Geometry: final body of the model. Coordinates: model frame, mm. A direction names the side the tool comes from. Give positions to 0.01 mm unless a question says otherwise; leave off trailing zeros. Loops run counter-clockwise (first coordinate to the right, second up) from the corner with the lowest first, then second, coordinate; pieces in that order, holes last. Notation, with made-up numbers: (82.25, 75.5) -> (97.25, 75.5) arc R26 ccw to (97.25, 106.5) -> close; hole circle Ø5 at (1.5, -26). An arc over 180 degrees is marked (long way). Answer in a Markdown table with one row per item. Add a question column.
1) Section query B-B (z = 32). Return the cut outline in (x, y) (3 decimals).
2) First-contact query: P1, Ø16.5, axis at y = 40.5, z = 17, coming from the -X side; P2, Ø24.5, axis at x = 254, y = 25.4, coming from the +Z side (3 decimals); P3, Ø5.5, axis at x = 416.33, y = 23.91, coming from the -Z side (3 decimals). Flat tips, straight axial feed; report the tip coordinate or a pass-through.
3) Section query C-C (x = 368.3). Return the cut outline in (y, z) (3 decimals).
4) Line query: line 1 (Y direction, x = 402, z = 21) (3 decimals); line 2 (Z direction, x = 243.5, y = 11) (3 decimals). Output: solid intervals per line, ascending. Write a range as from..to.
5) Access query for faces 5 (the flat face through (25.4, 48, 18)), 6 (the cylindrical face through (501.982, 31.504, 49.235)), 7 (the flat face through (363, 8, 0)). Directions: +Z, -Z, +X, -X, +Y, -Y. A direction counts if a zero-diameter tool reaches every point of the face in a straight line with its end or side. Return the directions, or none.
6) Draft query along Z for faces 1 (the flat face through (736.6, 48, 22)), 2 (the flat face through (363, 9, 50.8)), 3 (the flat face through (376, 47.625, 26)), 4 (the flat face through (379, 3.175, 25)). Return one class per face: +Z half, -Z half, draft (parallel to the pull), parting line (faces both ways), or undercut.
7) Section query A-A (x = 556). Return the cut outline in (y, z) (3 decimals), plus the area to 3 significant figures.
Autodesk Inventor part; units mm, degrees
ref_plane "YZ Plane" through (0, 0, 0) normal (1, 0, 0) x (0, 1, 0)
ref_plane "XZ Plane" through (0, 0, 0) normal (0, 1, 0) x (-1, 0, 0)
ref_plane "XY Plane" through (0, 0, 0) normal (0, 0, 1) x (1, 0, 0)
sketch "Sketch1" plane through (0, 0, 0) normal (1, 0, 0) x (0, 1, 0)
  line L0 (0, 0) -> (50.8, 0)
  line L1 (50.8, 0) -> (50.8, 50.8)
  line L2 (50.8, 50.8) -> (0, 50.8)
  line L3 (0, 50.8) -> (0, 0)
  line L4 (3.175, 47.625) -> (47.625, 47.625)
  line L5 (47.625, 47.625) -> (47.625, 3.175)
  line L6 (47.625, 3.175) -> (3.175, 3.175)
  line L7 (3.175, 3.175) -> (3.175, 47.625)
  dimension "d0" = 50.8
  dimension "d1" = 3.175
extrude "Extrusion1" add sketch "Sketch1" along normal blind 736.6
sketch "Sketch2" plane through (0, 0, 50.8) normal (0, 0, 1) x (1, 0, 0)
  line L0 (0, 50.8) -> (0, 0)
  line L1 (0, 0) -> (736.6, 0)
  line L2 (736.6, 50.8) -> (736.6, 0)
  line L3 (0, 50.8) -> (736.6, 50.8)
  circle A0 centre (48.0624, 26.9875) radius 14.2875
  circle A1 centre (368.3, 23.8125) radius 14.2875
  circle A2 centre (688.5376, 26.9875) radius 14.2875
  line L4 (-35.152, 25.4) -> (810.7598, 25.4) construction
  line L5 (736.6, 3.175) -> (736.6, 0)
  line L6 (736.6, 0) -> (733.425, 0)
  arc A3 (733.425, 0) -> (736.6, 3.175) centre (733.425, 3.175) ccw
  arc A4 (0, 25.4) -> (1.4704, 22.7214) centre (3.175, 25.4) ccw
  arc A5 (36.3954, 0.4964) -> (38.1, 0) centre (38.1, 3.175) ccw
  line L7 (1.4704, 22.7214) -> (36.3954, 0.4964)
  line L8 (0, 25.4) -> (0, 0)
  line L9 (38.1, 0) -> (0, 0)
  line L10 (-134.201, 26.9875) -> (938.3775, 26.9875) construction
  dimension "d4" = 25.4
  dimension "d5" = 23.8125
  dimension "d6" = 320.2534
  dimension "d7" = 320.2534
  dimension "d8" = 368.3
  dimension "d9" = 28.575
  dimension "d10" = 3.175
  dimension "d11" = 3.175
  dimension "d12" = 3.175
  dimension "d13" = 3.175
  dimension "d14" = 38.1
  dimension "d19" = 1.5875
extrude "Extrusion2" cut sketch "Sketch2" against normal blind 50.8 contours A4 L7 A5 L1 L0 | L2 L1 A3 | A0 | A1 | A2
sketch "Sketch3" plane through (736.6, 50.8, 0) normal (0, 0, -1) x (-1, 0, 0)
  line L0 (736.6, 0) -> (711.2, 0)
  line L1 (711.2, 0) -> (711.2, -25.4)
  line L2 (711.2, -25.4) -> (736.6, -25.4)
  line L3 (736.6, -25.4) -> (736.6, 0)
  line L4 (711.2, -25.4) -> (717.8505, -18.7495) construction
  circle A0 centre (713.4451, -23.1549) radius 3.175
  point P0 (736.6, -50.8)
  dimension "d24" = 6.35
  dimension "d17" = 25.4
  dimension "d22" = 45
extrude "Extrusion3" cut sketch "Sketch3" against normal blind 47.625
sketch "Sketch5" plane through (0, 50.8, 50.8) normal (0, 0, 1) x (1, 0, 0)
  line L0 (0, 0) -> (736.6, 0)
  line L1 (0, 0) -> (0, -25.4)
  circle A0 centre (368.3, -26.9875) radius 14.2875
  line L2 (-82.8733, -25.4) -> (895.8965, -25.4) construction
  circle A1 centre (127, -25.4) radius 20.32
  circle A2 centre (254, -25.4) radius 20.32
  circle A3 centre (482.6, -25.4) radius 20.32
  circle A4 centre (609.6, -25.4) radius 20.32
  point P0 (0, -50.8)
  dimension "d25" = 25.4
  dimension "d26" = 40.64
  dimension "d27" = 127
  dimension "d28" = 127
  dimension "d29" = 114.3
  dimension "d30" = 114.3
extrude "Extrusion4" cut sketch "Sketch5" against normal blind 3.175 contours A1 | A2 | A3 | A4
sketch "Sketch6" plane through (733.425, 0, 0) normal (0, 0, -1) x (-1, 0, 0)
  line L0 (733.425, 25.4) -> (712.5151, 25.4)
  circle A0 centre (365.125, 23.8125) radius 14.2875
  line L1 (217.4406, 23.9141) -> (492.0781, 23.9141) construction
  point P0 (733.425, 0)
  point P1 (432.3588, 23.9141)
  point P2 (344.424, 23.9141)
  point P3 (317.0936, 23.9141)
  dimension "d33" = 0.1016
  dimension "d34" = 20.701
  dimension "d35" = 48.0314
  dimension "d36" = 67.2338
hole "Hole1" at (301.0662, 23.9141, 0) at (389.001, 23.9141, 0) at (416.3314, 23.9141, 0) direction (0, 0, 1) diameter 7.9756 depth 25.4 tip angle 118
sketch "Sketch7" plane through (733.425, 0, 0) normal (0, 0, -1) x (-1, 0, 0)
  line L0 (733.425, 25.4) -> (712.5151, 25.4)
  circle A0 centre (365.125, 23.8125) radius 14.2875
  line L1 (252.4125, 28.8925) -> (487.3625, 28.8925) construction
  point P0 (733.425, 0)
  point P1 (307.5686, 28.8925)
  point P2 (441.8838, 28.8925)
  dimension "d44" = 5.08
  dimension "d45" = 57.5564
  dimension "d46" = 76.7588
hole "Hole2" at (425.8564, 28.8925, 0) at (291.5412, 28.8925, 0) direction (0, 0, 1) diameter 6.35 depth 25.4 tip angle 118
sketch "Sketch8" plane through (0, 50.8, 50.8) normal (0, 0, 1) x (1, 0, 0)
  circle A0 centre (482.6, -25.4) radius 20.32
  circle A1 centre (127, -25.4) radius 20.32
  circle A2 centre (254, -25.4) radius 20.32
  circle A3 centre (609.6, -25.4) radius 20.32
  arc A4 (36.3954, -50.3036) -> (38.1, -50.8) centre (38.1, -47.625) ccw
  line L0 (38.1, -50.8) -> (733.425, -50.8)
  arc A5 (733.425, -50.8) -> (736.6, -47.625) centre (733.425, -47.625) ccw
  line L1 (736.6, 0) -> (736.6, -47.625)
  line L2 (0, 0) -> (736.6, 0)
  line L3 (0, 0) -> (0, -25.4)
  arc A6 (0, -25.4) -> (1.4704, -28.0786) centre (3.175, -25.4) ccw
  line L4 (1.4704, -28.0786) -> (36.3954, -50.3036)
  circle A7 centre (368.3, -26.9875) radius 14.2875
  circle A8 centre (48.0624, -23.8125) radius 14.2875
  circle A9 centre (688.5376, -23.8125) radius 14.2875
  circle A10 centre (291.5412, -21.9075) radius 3.175
  circle A11 centre (301.0662, -26.8859) radius 3.9878
  circle A12 centre (389.001, -26.8859) radius 3.9878
  circle A13 centre (416.3314, -26.8859) radius 3.9878
  circle A14 centre (425.8564, -21.9075) radius 3.175
  point P0 (0, -50.8)
hole "Hole3" at (301.0662, 23.9141, 50.8) at (389.001, 23.9141, 50.8) at (416.3314, 23.9141, 50.8) direction (0, 0, -1) diameter 4.7625 depth 25.4 tip angle 118
sketch "Sketch9" plane through (0, 50.8, 50.8) normal (0, 0, 1) x (1, 0, 0)
  circle A0 centre (291.5412, -21.9075) radius 3.175
  circle A1 centre (425.8564, -21.9075) radius 3.175
  point P0 (0, -50.8)
hole "Hole4" at (291.5412, 28.8925, 50.8) at (425.8564, 28.8925, 50.8) direction (0, 0, -1) diameter 9.525 depth 25.4 tip angle 118
sketch "Sketch11" plane through (733.425, 0, 0) normal (0, 0, -1) x (-1, 0, 0)
  circle A0 centre (307.5686, 28.8925) radius 3.175
  circle A1 centre (441.8838, 28.8925) radius 3.175
  circle A2 centre (344.424, 23.9141) radius 3.9878
  circle A3 centre (432.3588, 23.9141) radius 3.9878
  circle A4 centre (317.0936, 23.9141) radius 3.9878
  line L0 (708.025, 29.8901) -> (708.025, 50.8)
  line L1 (708.025, 50.8) -> (-3.175, 50.8)
  line L2 (-3.175, 3.175) -> (-3.175, 50.8)
  arc A5 (-3.175, 3.175) -> (0, 0) centre (0, 3.175) ccw
  line L3 (695.325, 0) -> (0, 0)
  arc A6 (695.325, 0) -> (697.0296, 0.4964) centre (695.325, 3.175) ccw
  line L4 (697.0296, 0.4964) -> (731.9546, 22.7214)
  arc A7 (731.9546, 22.7214) -> (733.425, 25.4) centre (730.25, 25.4) ccw
  line L5 (733.425, 25.4) -> (712.5151, 25.4)
  arc A8 (708.025, 29.8901) -> (712.5151, 25.4) centre (710.2701, 27.6451) ccw
  circle A9 centre (365.125, 23.8125) radius 14.2875
  circle A10 centre (685.3626, 26.9875) radius 14.2875
  circle A11 centre (44.8874, 26.9875) radius 14.2875
  point P0 (733.425, 0)
sketch "Sketch12" plane through (733.425, 0, 0) normal (0, 0, -1) x (-1, 0, 0)
  circle A0 centre (307.5686, 28.8925) radius 3.175
  circle A1 centre (441.8838, 28.8925) radius 3.175
  circle A2 centre (344.424, 23.9141) radius 3.9878
  circle A3 centre (432.3588, 23.9141) radius 3.9878
  circle A4 centre (317.0936, 23.9141) radius 3.9878
  line L0 (708.025, 29.8901) -> (708.025, 50.8)
  line L1 (708.025, 50.8) -> (-3.175, 50.8)
  line L2 (-3.175, 3.175) -> (-3.175, 50.8)
  arc A5 (-3.175, 3.175) -> (0, 0) centre (0, 3.175) ccw
  line L3 (695.325, 0) -> (0, 0)
  arc A6 (695.325, 0) -> (697.0296, 0.4964) centre (695.325, 3.175) ccw
  line L4 (697.0296, 0.4964) -> (731.9546, 22.7214)
  arc A7 (731.9546, 22.7214) -> (733.425, 25.4) centre (730.25, 25.4) ccw
  line L5 (733.425, 25.4) -> (712.5151, 25.4)
  arc A8 (708.025, 29.8901) -> (712.5151, 25.4) centre (710.2701, 27.6451) ccw
  circle A9 centre (365.125, 23.8125) radius 14.2875
  circle A10 centre (685.3626, 26.9875) radius 14.2875
  circle A11 centre (44.8874, 26.9875) radius 14.2875
  line L6 (713.7121, 11.1125) -> (756.5701, 38.3858)
  line L7 (733.425, 25.4) -> (733.425, 4.1402)
  line L8 (695.325, 0) -> (700.957, 0)
  line L9 (713.7121, 11.1125) -> (685.3626, -6.9281)
  line L10 (733.425, 23.6571) -> (740.2433, 12.9426)
  line L11 (696.2496, 0) -> (703.0679, -10.7145)
  line L12 (740.2433, 12.9426) -> (733.425, 12.9426)
  line L13 (703.0679, -10.7145) -> (703.0679, 0)
  line L14 (703.0679, 0) -> (696.2496, 0)
  point P0 (733.425, 0)
  dimension "d69" = 12.7
  dimension "d70" = 12.7
  dimension "d71" = 10.7145
  dimension "d72" = 6.8183
  dimension "d75" = 6.8183
  dimension "d76" = 37.1754
  dimension "d77" = 23.6571
equation "\"d7\" = d6"
equation "\"d11\" = d10"
equation "\"d13\" = d12"
equation "\"d28\" = d27"
equation "\"d30\" = d29"
properties part number "RightMainBeam" material "Aluminum 6061"
Evaluation:
| question | item | result |
|---|---|---|
| 1 | outline | (25.4, 47.625) -> (736.6, 47.625) -> (736.6, 50.8) -> (25.4, 50.8) -> close; (32.186, 3.175) -> (36.395, 0.496) arc R3.175 ccw to (38.1, 0) -> (733.425, 0) arc R3.175 ccw to (736.6, 3.175) -> close |
| 2 | P1 | x = 25.4 |
| 2 | P2 | z = 3.175 |
| 2 | P3 | z = 47.625 |
| 3 | outline | (0, 0) -> (9.525, 0) -> (9.525, 3.175) -> (3.175, 3.175) -> (3.175, 47.625) -> (9.525, 47.625) -> (9.525, 50.8) -> (0, 50.8) -> close; (38.1, 0) -> (50.8, 0) -> (50.8, 50.8) -> (38.1, 50.8) -> (38.1, 47.625) -> (47.625, 47.625) -> (47.625, 3.175) -> (38.1, 3.175) -> close |
| 4 | line 1 | 0..3.175, 47.625..50.8 |
| 4 | line 2 | 0..3.175 |
| 5 | face 5 | -Z, -X, +Y |
| 5 | face 6 | +Z |
| 5 | face 7 | -Z, +X, -X, +Y, -Y |
| 6 | face 1 | draft |
| 6 | face 2 | +Z half |
| 6 | face 3 | undercut |
| 6 | face 4 | undercut |
| 7 | outline | (0, 0) -> (50.8, 0) -> (50.8, 50.8) -> (0, 50.8) -> close; hole (3.175, 3.175) -> (47.625, 3.175) -> (47.625, 47.625) -> (3.175, 47.625) -> close |
| 7 | area | 605 mm² |
